Design review of the part built by this model. Coordinates are the model's own, in mm. A direction names the side the tool comes from. Give positions to 0.01 mm unless a question says otherwise; leave off trailing zeros. Write each loop counter-clockwise with the first axis right and the second up, starting at its lowest first coordinate (ties: lowest second). Pieces come first, ordered by that corner, then holes.
```python
from build123d import *

# Parameters (mm, degrees)
BOSS_EXTRUDE1_DEPTH      = 11.2
BOSS_EXTRUDE1_DEPTH_BACK = 11.2
CUT_EXTRUDE1_START       = -11.2
SKETCH3_R                = 7.5
CUT_EXTRUDE1_DEPTH       = 22.4
FILLET1_R                = 10
CUT_EXTRUDE2_START       = -11.2
CUT_EXTRUDE2_DEPTH       = 22.4
FILLET2_R                = 10
BOSS_EXTRUDE2_START      = -11.2
BOSS_EXTRUDE2_DEPTH      = 22.4
FILLET3_R                = 10
CUT_EXTRUDE3_START       = -11.2
CUT_EXTRUDE3_DEPTH       = 22.4
CUT_EXTRUDE4_START       = -11.2
SKETCH7_R                = 3
CUT_EXTRUDE4_DEPTH       = 22.4


with BuildPart() as part:
    # Sketch2 → Boss-Extrude1 (new, two sides: drawn at the far end of the back side and taken through both)
    with BuildSketch(Plane(origin=(0, 0, 0), x_dir=(0, 0, -1), z_dir=(1, 0, 0)).offset(-BOSS_EXTRUDE1_DEPTH_BACK)):
        with BuildLine():
            Line((-52.85, 26.5), (32.85, 26.5))
            ThreePointArc((32.85, 26.5), (52.85, 0), (32.85, -26.5))
            Line((32.85, -26.5), (-40.85, -26.5))
            ThreePointArc((-40.85, -26.5), (-49.335281374, -22.985281374), (-52.85, -14.5))
            Line((-52.85, -14.5), (-52.85, 26.5))
        make_face()
        with BuildLine():
            Line((32.85, 20.5), (-40.85, 20.5))
            ThreePointArc((-40.85, 20.5), (-45.092640687, 18.742640687), (-46.85, 14.5))
            Line((-46.85, 14.5), (-46.85, -8.5))
            ThreePointArc((-46.85, -8.5), (-43.335281374, -16.985281374), (-34.85, -20.5))
            Line((-34.85, -20.5), (32.85, -20.5))
            ThreePointArc((32.85, -20.5), (47.142020276, 0), (32.85, 20.5))
        make_face(mode=Mode.SUBTRACT)
    extrude(amount=BOSS_EXTRUDE1_DEPTH + BOSS_EXTRUDE1_DEPTH_BACK)

    # Sketch3 → Cut-Extrude1 (cut)
    with BuildSketch(Plane(origin=(0, 0, 0), x_dir=(0, 0, -1), z_dir=(1, 0, 0)).offset(CUT_EXTRUDE1_START)):
        with Locations((-40.85, 14.5)):
            Circle(SKETCH3_R)
        with Locations((-20.85, 14.5)):
            Circle(SKETCH3_R)
        with Locations((-0.85, 14.5)):
            Circle(SKETCH3_R)
        with Locations((19.15, 14.5)):
            Circle(SKETCH3_R)
    extrude(amount=CUT_EXTRUDE1_DEPTH, mode=Mode.SUBTRACT)

    # Fillet1
    fillet1_edges = [part.edges().sort_by_distance(p)[0] for p in [
        (0, 20.5, -32.85),
    ]]
    fillet(fillet1_edges, radius=FILLET1_R)

    # Sketch4 → Cut-Extrude2 (cut)
    with BuildSketch(Plane(origin=(0, 0, 0), x_dir=(0, 0, -1), z_dir=(1, 0, 0)).offset(CUT_EXTRUDE2_START)):
        Polygon((-46.85, -8.5), (-48.333754922, 14.006631719), (-46.85, 14.006631719), align=None)
    extrude(amount=CUT_EXTRUDE2_DEPTH, mode=Mode.SUBTRACT)

    # Fillet2
    fillet2_edges = [part.edges().sort_by_distance(p)[0] for p in [
        (0, -20.5, -32.85),
        (0, 26.5, -32.85),
        (0, -26.5, -32.85),
    ]]
    fillet(fillet2_edges, radius=FILLET2_R)

    # Sketch5 → Boss-Extrude2 (add)
    with BuildSketch(Plane(origin=(0, 0, 0), x_dir=(0, 0, -1), z_dir=(1, 0, 0)).offset(BOSS_EXTRUDE2_START)):
        with BuildLine():
            Line((-52.85, -6.3), (-52.85, 26.5))
            Line((-52.85, 26.5), (-82.85, 26.5))
            Line((-82.85, 26.5), (-82.85, 28.5))
            ThreePointArc((-82.85, 28.5), (-84.314466094, 32.035533906), (-87.85, 33.5))
            Line((-87.85, 33.5), (-92.85, 33.5))
            ThreePointArc((-92.85, 33.5), (-96.385533906, 32.035533906), (-97.85, 28.5))
            Line((-97.85, 28.5), (-97.85, 26.5))
            Line((-97.85, 26.5), (-79.85, -19.82922762))
            ThreePointArc((-79.85, -19.82922762), (-64.75, -16.257700748), (-52.85, -6.3))
        make_face()
    extrude(amount=BOSS_EXTRUDE2_DEPTH)

    # Fillet3
    fillet3_edges = [part.edges().sort_by_distance(p)[0] for p in [
        (0, -19.82922762, 79.85),
    ]]
    fillet(fillet3_edges, radius=FILLET3_R)

    # Sketch6 → Cut-Extrude3 (cut)
    with BuildSketch(Plane(origin=(0, 0, 0), x_dir=(0, 0, -1), z_dir=(1, 0, 0)).offset(CUT_EXTRUDE3_START)):
        with BuildLine():
            Line((-53.333754922, 14.006631719), (-53.333754922, 1.506631719))
            ThreePointArc((-53.333754922, 1.506631719), (-58.833754922, -3.993368281), (-64.333754922, 1.506631719))
            Line((-64.333754922, 1.506631719), (-64.333754922, 14.006631719))
            ThreePointArc((-64.333754922, 14.006631719), (-58.833754922, 19.506631719), (-53.333754922, 14.006631719))
        make_face()
    extrude(amount=CUT_EXTRUDE3_DEPTH, mode=Mode.SUBTRACT)

    # Sketch7 → Cut-Extrude4 (cut)
    with BuildSketch(Plane(origin=(0, 0, 0), x_dir=(0, 0, -1), z_dir=(1, 0, 0)).offset(CUT_EXTRUDE4_START)):
        with Locations((-90.35, 26.5)):
            Circle(SKETCH7_R)
    extrude(amount=CUT_EXTRUDE4_DEPTH, mode=Mode.SUBTRACT)


solid = part.part
```
(1) Consider section D-D, the plane z = 63. Give the boundary of the cut face in (x, y).
Resolved:
outline: (-11.2, -15.32) - (11.2, -15.32) - (11.2, -2.08) - (-11.2, -2.08) - close; (-11.2, 17.6) - (11.2, 17.6) - (11.2, 26.5) - (-11.2, 26.5) - close
(2) Mouldability with a two-part tool opening along Z and no side actions: class faces 1 (the face through (0, 20.5, 31)), 2 (the face through (0, 33.5, 90)), 3 (the face through (-0.16, 32, 84.28)) as pulls with the +Z half, pulls with the -Z half, needs draft (parallel to the pull), parting line crosses it, or undercut.
Resolved:
face 1: undercut
face 2: needs draft
face 3: pulls with the -Z half
(3) Consider section B-B, the plane x = 1.25. Give the number of separate pieces and of enclosed holes in the cut face, then the cut area to 3 significant figures.
Resolved:
separate pieces: 1
enclosed holes: 3
area: 2,950 mm2
(4) Consider section A-A, the plane z = -13. Give the boundary of the cut face in (x, y).
Resolved:
outline: (-11.2, -26.5) - (11.2, -26.5) - (11.2, -20.5) - (-11.2, -20.5) - close; (-11.2, 20.5) - (11.2, 20.5) - (11.2, 26.5) - (-11.2, 26.5) - close
(5) Clearance check with flat-ended pins moving along their axes: P1, Ø3, axis at x = -4.5, y = -18, coming from the +Z side; P2, Ø6, axis at x = -4.5, y = 3, coming from the +Z side; P3, Ø8, axis at x = 3.5, y = -8, coming from the -Z side; P4, Ø8, axis at x = 6.5, y = -2.5, coming from the -Z side. State where each tip first meets the part, or that it passes through.
Resolved:
P1: stops at z = 79.89
P2: stops at z = 89.89
P3: stops at z = -52.56
P4: stops at z = -52.85
(6) Tool access review of faces 4 (the face through (0.157, -17.923, 77.718)), 5 (the face through (0, 26.5, 25)), 6 (the face through (0, 20.5, 11)): name each direction out of +Z, -Z, +X, -X, +Y, -Y from which nothing blocks a thin tool from reaching the whole face with its end or side.
Resolved:
face 4: +X, -X, -Y
face 5: -Z, +X, -X, +Y
face 6: +X, -X
(7) Consider section C-C, the plane y = 16.5. Give the boundary of the cut face in (x, z).
Resolved:
outline: (-11.2, -47.36) - (11.2, -47.36) - (11.2, -39.61) - (-11.2, -39.61) - close; (-11.2, 48.08) - (11.2, 48.08) - (11.2, 53.93) - (-11.2, 53.93) - close; (-11.2, 63.74) - (11.2, 63.74) - (11.2, 93.96) - (-11.2, 93.96) - close
(8) To check wall thickness, follow L1, parallel to Y at x = -1.25, z = -19; L2, parallel to Y at x = 4.5, z = -14; L3, parallel to Z at x = 0.75, y = -14.5. State the ranges of each line that lie inside material, in increasing order.
Resolved:
L1: y = -26.5 to -20.5, 22 to 26.5
L2: y = -26.5 to -20.5, 20.5 to 26.5
L3: z = -48.73 to -41.64, 45.24 to 52.85, 61.66 to 81.66
